Build history of the part. All positions in model axes, mm. Face numbers are marked on the shaded views. A direction names the side the tool comes from. Give positions to 0.01 mm unless a question says otherwise; leave off trailing zeros. Write each loop counter-clockwise with the first axis right and the second up, starting at its lowest first coordinate (ties: lowest second). Pieces come first, ordered by that corner, then holes. Notation, with made-up numbers: (41, 29.5) -> (96, 29.5) arc R30 ccw to (96, 68.5) -> close; hole circle Ø10 at (-20, -30.75). An arc over 180 degrees is marked (long way). Write item = value, one per line. Start each with the question number.
Q1. Saw through at B-B, the plane x = -20. List the corners of the cut face in (y, z).
Q2. Saw through at C-C, the plane z = 5.5. List the corners of the cut face in (x, y).
Q3. Saw through at A-A, the plane y = 12. List the corners of the cut face in (x, z), then the cut area to 3 significant figures.
Q4. Tool access for the marked faces 1 and 2: list every direction of +Z, -Z, +X, -X, +Y, -Y with a clear straight run to the whole face (end or side of a thin tool).
Q5. Wall check: line 1 (Z direction, x = 20, y = 3.15); line 2 (X direction, y = 0.5, z = 2.5) (3 decimals); line 3 (Y direction, x = 20, z = -1). Give the ranges that are in metal, low to high.
Q6. Saw through at D-D, the plane y = 1. Give the number of separate pieces and of enclosed holes in the cut face, then the cut area to 3 significant figures.
Q7. Mould opens along X. For the marked faces 3, 4 and 5 say: pulls with the +X half, pulls with the -X half, needs draft (parallel to the pull), parting line crosses it, or undercut.
Q8. Drop flat-ended pins along their axis: P1, Ø1.2, axis at x = -13.5, y = 3, coming from the -Z side; P2, Ø6, axis at y = 14, z = 8.5, coming from the -X side; P3, Ø3, axis at x = -6.5, y = 11.5, coming from the +Z side; P4, Ø2, axis at y = -2.5, z = 1.5, coming from the +X side. Give the stop position or say it passes through.
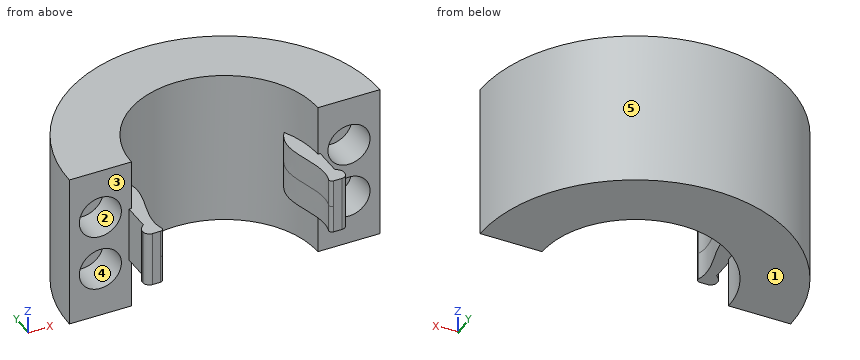
from build123d import *

# Parameters (mm, degrees)
BOSS_EXTRUDE1_DEPTH = 12.5
BOSS_EXTRUDE3_DEPTH = 4.42775
FILLET1_R           = 1
FILLET2_R           = 1
FILLET5_R           = 1
FILLET6_R           = 1
SKETCH4_R           = 3.388
CUT_EXTRUDE1_DEPTH  = 5.656
FILLET7_R           = 0.5


with BuildPart() as part:
    # Sketch1 → Boss-Extrude1 (new body, symmetric)
    with BuildSketch(Plane.XY):
        with BuildLine():
            Line((-25, 0), (-15, 0))
            ThreePointArc((-15, 0), (0, 15), (15, 0))
            Line((15, 0), (25, 0))
            ThreePointArc((25, 0), (0, 25), (-25, 0))
        make_face()
    extrude(amount=BOSS_EXTRUDE1_DEPTH, both=True)

    # Sketch3 → Boss-Extrude3 (add, symmetric)
    with BuildSketch(Plane.XY):
        with BuildLine():
            Line((15.3827, 0), (15.3827, -4.45))
            Line((15.3827, -4.45), (16.2282, -5.2955))
            Line((16.2282, -5.2955), (16.2282, -7.031))
            Line((16.2282, -7.031), (13.2022, -7.031))
            add(Edge.make_bspline(
                [(13.2022, 7.12052773), (9.986819902, 2.44993192), (15.309996934, -2.18235212), (13.2022, -7.031)],
                knots=[0, 0, 0, 0, 1, 1, 1, 1], degree=3))
            ThreePointArc((13.2022, 7.12052773), (14.543606843, 3.671988562), (15, 0))
            Line((15, 0), (15.3827, 0))
        make_face()
    boss_extrude3 = extrude(amount=BOSS_EXTRUDE3_DEPTH, both=True)

    # Mirror11: Boss-Extrude3 across plane
    add(boss_extrude3.mirror(Plane(origin=(0, 0, 0), x_dir=(0, 0, 1), z_dir=(1, 0, 0))))

    # Fillet1
    fillet1_edges = [part.edges().sort_by_distance(p)[0] for p in [
        (16.2282, -7.031, 0),
    ]]
    fillet(fillet1_edges, radius=FILLET1_R)

    # Fillet2
    fillet2_edges = [part.edges().sort_by_distance(p)[0] for p in [
        (-16.2282, -7.031, 0),
    ]]
    fillet(fillet2_edges, radius=FILLET2_R)

    # Fillet5
    fillet5_edges = [part.edges().sort_by_distance(p)[0] for p in [
        (16.2282, -5.2955, 0),
    ]]
    fillet(fillet5_edges, radius=FILLET5_R)

    # Fillet6
    fillet6_edges = [part.edges().sort_by_distance(p)[0] for p in [
        (-16.2282, -5.2955, 0),
    ]]
    fillet(fillet6_edges, radius=FILLET6_R)

    # Sketch4 → Cut-Extrude1 (cut)
    with BuildSketch(Plane.XZ):
        with Locations((20, -4.5)):
            Circle(SKETCH4_R)
        with Locations((20, 4.5)):
            Circle(SKETCH4_R)
    cut_extrude1 = extrude(amount=-CUT_EXTRUDE1_DEPTH, mode=Mode.SUBTRACT)

    # Mirror12: Cut-Extrude1 across plane
    add(cut_extrude1.mirror(Plane(origin=(0, 0, 0), x_dir=(0, 0, 1), z_dir=(1, 0, 0))), mode=Mode.SUBTRACT)

    # Fillet7
    fillet7_edges = [part.edges().sort_by_distance(p)[0] for p in [
        (13.2022, -7.031, 2.213875),
        (-13.2022, -7.031, -2.213875),
    ]]
    fillet(fillet7_edges, radius=FILLET7_R)


solid = part.part
Report:
q1.outline = (0, -12.5) -> (15, -12.5) -> (15, 12.5) -> (0, 12.5) -> (0, 7.89) -> (5.66, 7.89) -> (5.66, 1.11) -> (0, 1.11) -> (0, -1.11) -> (5.66, -1.11) -> (5.66, -7.89) -> (0, -7.89) -> close
q2.outline = (-25, 0) -> (-23.24, 0) -> (-23.24, 5.66) -> (-16.76, 5.66) -> (-16.76, 0) -> (-15, 0) arc R15 cw to (15, 0) -> (16.76, 0) -> (16.76, 5.66) -> (23.24, 5.66) -> (23.24, 0) -> (25, 0) arc R25 ccw to start
q3.outline = (-21.93, -12.5) -> (-9, -12.5) -> (-9, 12.5) -> (-21.93, 12.5) -> close; (9, -12.5) -> (21.93, -12.5) -> (21.93, 12.5) -> (9, 12.5) -> close
q3.area = 647 mm2
q4.face_1 = -Z, +X, -X, +Y, -Y
q4.face_2 = -Y
q5.line_1 = -12.5 to -7.89, -1.11 to 1.11, 7.89 to 12.5
q5.line_2 = -24.995 to -22.735, -17.265 to -12.678, 12.678 to 17.265, 22.735 to 24.995
q5.line_3 = 0 to 15
q6.separate_pieces = 2
q6.enclosed_holes = 4
q6.area = 399 mm2
q7.face_3 = needs draft
q7.face_4 = undercut
q7.face_5 = parting line crosses it
q8.P1 = -4.43
q8.P2 = -22.45
q8.P3 = through
q8.P4 = 15.38
